Source: three-view drawing plus pictorial views. Frame: mm from the lowest corner of the part. Round coordinates to 2 decimals unless told otherwise and drop trailing zeros. Write each loop counter-clockwise with the first axis right and the second up, starting at its lowest first coordinate (ties: lowest second). Pieces come first, ordered by that corner, then holes. Notation, with made-up numbers: (77, -23) - (136, -23) arc R37 cw to (136, 15) - close; hole circle Ø4 at (47.5, -20). An arc over 180 degrees is marked (long way). Write each question's results on one line, items separated by ' | '.
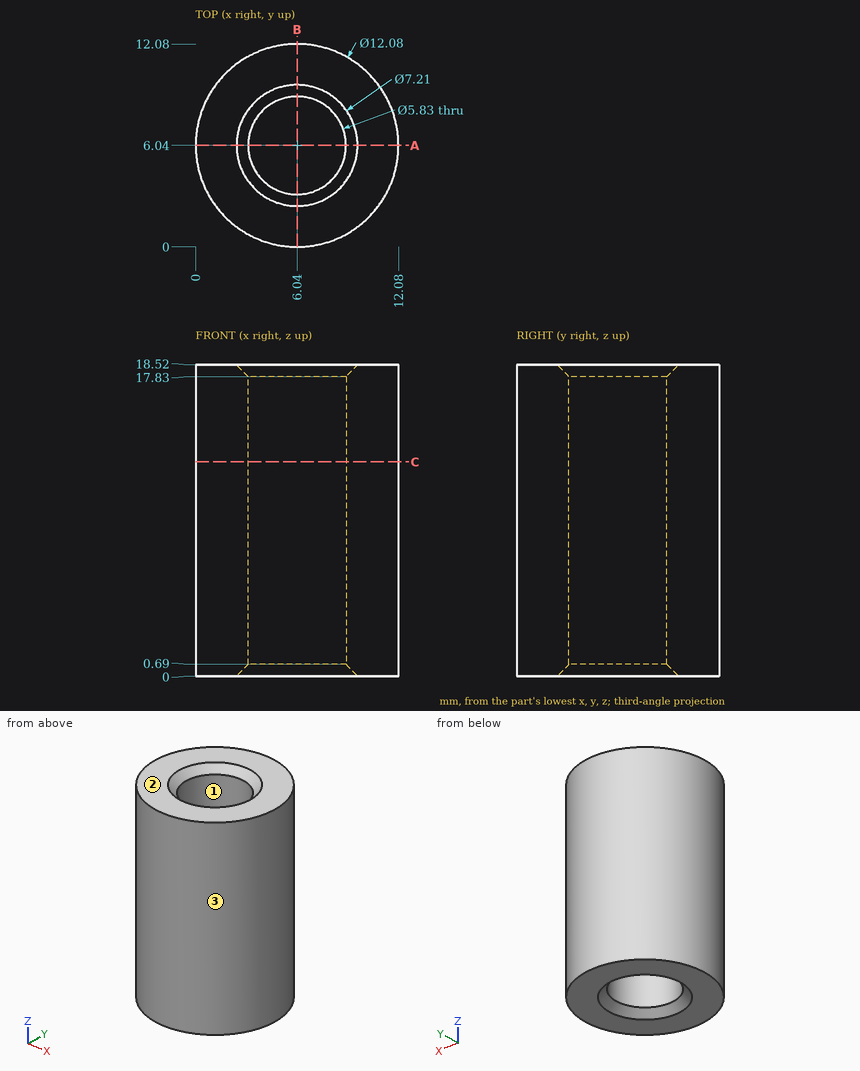
Q1. Mould query, pull axis Y, two halves, no side actions, for the marked faces 1, 2 and 3. Classes: pulls with the +Y half, pulls with the -Y half, needs draft (parallel to the pull), parting line crosses it, or undercut.
Answer block:
face 1: undercut | face 2: needs draft | face 3: parting line crosses it
Q2. Section query C-C, the plane z = 12.75. Return loops of the section in (x, y) (3 decimals), plus the area to 3 significant figures.
Answer block:
outline: circle Ø12.08 at (6.04, 6.04); hole circle Ø5.83 at (6.04, 6.04) | area: 87.9 mm2
Q3. Pin query (flat end, axial travel): pin 1 (3 mm diameter, centred on x = 3.5, z = 11, fed in from -Y); pin 2 (2 mm diameter, centred on x = 2.5, z = 13, fed in from +Y); pin 3 (1.5 mm diameter, centred on x = 5.5, y = 1.5, fed in from -Z); pin 4 (4 mm diameter, centred on y = 8.5, z = 6.5, fed in from +X). Return the tip coordinate at first contact, or that it passes through.
Answer block:
pin 1: y = 0.09 | pin 2: y = 11.52 | pin 3: z = 0 | pin 4: x = 12.06
Q4. Section query A-A, the plane y = 6.04. Return loops of the section in (x, z) (3 decimals), plus the area to 3 significant figures.
Answer block:
outline: (0, 0) - (2.435, 0) - (3.125, 0.69) - (3.125, 17.83) - (2.435, 18.52) - (0, 18.52) - close; (8.955, 0.69) - (9.645, 0) - (12.08, 0) - (12.08, 18.52) - (9.645, 18.52) - (8.955, 17.83) - close | area: 115 mm2
Q5. Ray query, line 1 along X through (y, z) = (6, 7); line 2 along Y through (x, z) = (6.04, 4.5) (3 decimals). Return the intervals inside material, ascending.
Answer block:
line 1: 0 to 3.13, 8.95 to 12.08 | line 2: 0 to 3.125, 8.955 to 12.08
